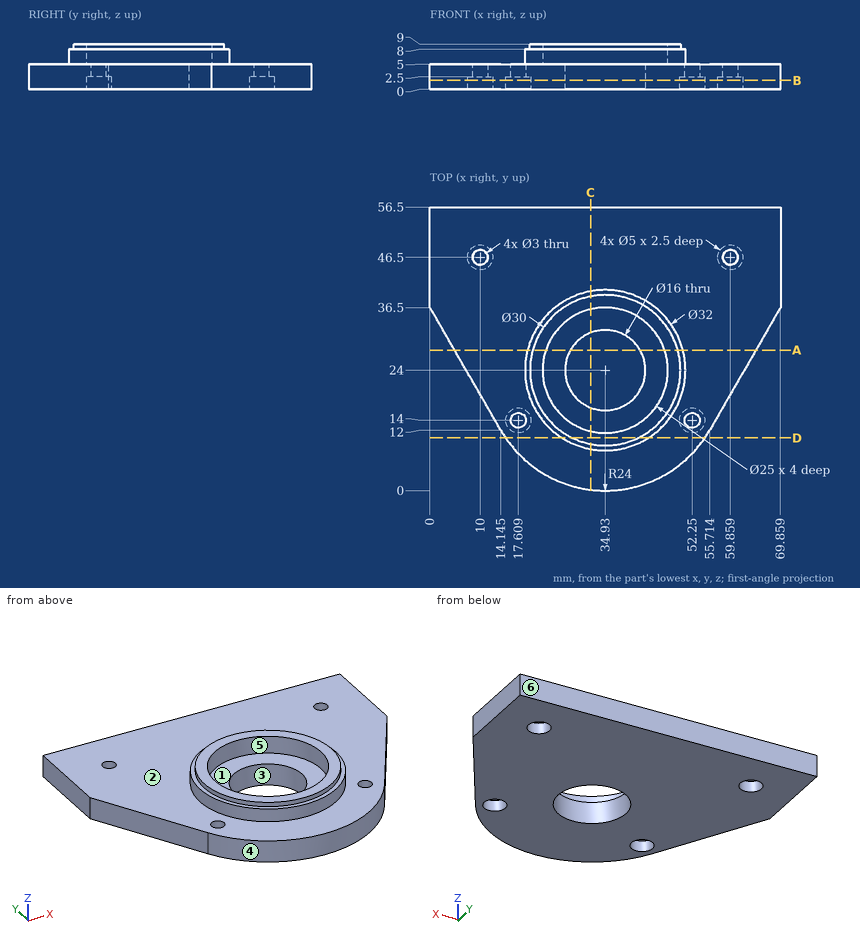
For this review, use the dimensioned drawing (mm, ordinates from the lowest corner) and the shaded views. A direction names the side the tool comes from. Round coordinates to 2 decimals unless told otherwise and drop trailing zeros. Order: outer loops, then holes, each group sorted by start corner. A loop starts at its lowest first (then second) coordinate and runs counter-clockwise, first axis right, second up. Notation, with made-up numbers: (-38, -30) -> (11, -30) arc R5 ccw to (11, -23) -> close; hole circle Ø9 at (0.5, 48.5). An arc over 180 degrees is marked (long way). One line per item, written item: value. Start each with the question number.
Q1. Take a section at B-B (z = 1.75). Count the separate pieces of the cut face and the enclosed holes in it, and give its area (3 significant figures).
Q2. Wall thickness on line 1 (X direction, y = 46.5, z = 4.45); line 2 (X direction, y = 13.5, z = 2.75) (1 decimal); line 3 (Z direction, x = 27, y = 9.5): over which ranges is each line inside the solid? List them lowest first.
Q3. Clearance check with flat-ended pins moving along their axes: pin 1 Ø2.5 at (x, y) = (17.5, 14.5) entering from -Z; pin 2 Ø12 at (x, y) = (7, 9) entering from -Z; pin 3 Ø6 at (x, y) = (52.25, 14) entering from -Z; pin 4 Ø4 at (x, y) = (52.25, 14) entering from +Z. State where each tip first meets the part, or that it passes through.
Q4. Mouldability with a two-part tool opening along Y and no side actions: class the marked faces 1, 2, 3 and 4 as released by +Y, released by -Y, zero draft, split by the parting line, or undercut.
Q5. Take a section at D-D (y = 10.5). Write out the cut boundary in (x, z), and give its area (3 significant figures).
Q6. Take a section at A-A (y = 28). Write out the cut boundary in (x, z), and give its area (3 significant figures).
Q7. Take a section at C-C (x = 32). Write out the cut boundary in (y, z) (1 decimal).
Q8. Machinability: for the marked faces 5 and 6, which of the approach directions +Z, -Z, +X, -X, +Y, -Y give a long, thin tool a straight path to every point of the face, cutting with its end or side? Answer none if there is none.
Reported:
1. separate pieces: 1
1. enclosed holes: 5
1. area: 2,840 mm2
2. line 1: x = 0 to 8.5, 11.5 to 58.36, 61.36 to 69.86
2. line 2: x = 13.3 to 16.2, 19 to 50.8, 53.7 to 56.6
2. line 3: z = 0 to 5
3. pin 1: stops at z = 2.5
3. pin 2: passes through
3. pin 3: stops at z = 0
3. pin 4: stops at z = 5
4. face 1: undercut
4. face 2: zero draft
4. face 3: undercut
4. face 4: released by -Y
5. outline: (15.09, 0) -> (54.77, 0) -> (54.77, 5) -> (43.52, 5) -> (43.52, 8) -> (41.47, 8) -> (41.47, 9) -> (28.39, 9) -> (28.39, 8) -> (26.34, 8) -> (26.34, 5) -> (15.09, 5) -> close
5. area: 263 mm2
6. outline: (4.91, 0) -> (28, 0) -> (28, 5) -> (23.09, 5) -> (23.09, 9) -> (20.47, 9) -> (20.47, 8) -> (19.44, 8) -> (19.44, 5) -> (4.91, 5) -> close; (41.86, 0) -> (64.95, 0) -> (64.95, 5) -> (50.42, 5) -> (50.42, 8) -> (49.39, 8) -> (49.39, 9) -> (46.77, 9) -> (46.77, 5) -> (41.86, 5) -> close
6. area: 258 mm2
7. outline: (0.2, 0) -> (16.6, 0) -> (16.6, 5) -> (11.8, 5) -> (11.8, 9) -> (9.3, 9) -> (9.3, 8) -> (8.3, 8) -> (8.3, 5) -> (0.2, 5) -> close; (31.4, 0) -> (56.5, 0) -> (56.5, 5) -> (39.7, 5) -> (39.7, 8) -> (38.7, 8) -> (38.7, 9) -> (36.2, 9) -> (36.2, 5) -> (31.4, 5) -> close
8. face 5: +Z
8. face 6: +Z, -Z, +X, -X, +Y
